Geometry check sheet. Reference: the model listing, model coordinates, mm. A direction names the side the tool comes from. Give positions to 0.01 mm unless a question says otherwise; leave off trailing zeros. Write each loop counter-clockwise with the first axis right and the second up, starting at its lowest first coordinate (ties: lowest second). Pieces come first, ordered by that corner, then holes. Notation, with made-up numbers: (-18, 81.5) - (37, 81.5) arc R10 cw to (37, 89.5) - close; hole circle Ø10 at (-37.75, -36.75). An arc over 180 degrees is marked (long way). Write item = value, one per line. Start each with the question number.
(1) Access from +Z, -Z, +X, -X, +Y, -Y to the whole of each face (thin tool, end or side, straight path). Record for faces 1 (the flat face through (-99, 1, 457.2)), 2 (the cylindrical face through (-62.084, 11.444, 392.811)).
(2) Section check C-C, the plane z = 399. Enter the section's corners in (x, y) (3 decimals), plus the area to 3 significant figures.
(3) Depth check by flat-ended pin: pin 1 Ø12 at (x, z) = (4, 264.5) entering from +Y; pin 2 Ø2 at (x, y) = (11.5, 147.5) entering from +Z; pin 3 Ø1.5 at (x, z) = (-137.5, 60.5) entering from +Y. Enter the tip coordinate at first touch or a pass-through.
(4) Section check A-A, the plane y = 0. Enter the section's corners in (x, z) (3 decimals), plus the area to 3 significant figures.
(5) Section check B-B, the plane x = 44.45. Enter the section's corners in (y, z), plus the area to 3 significant figures.
(6) Section check D-D, the plane z = 217.5. Enter the section's corners in (x, y).
(7) Thickness scan on L1, parallel to Z at x = 76, y = -124.5; L2, parallel to X at y = -14, z = 299.5; L3, parallel to Y at x = 138.5, z = 310.5. Record the ranges inside material, lowest first.
```python
from build123d import *

# Parameters (mm, degrees)
F1_DEPTH = 330.2
F2_R     = 38.1
F3_DEPTH = 127


with BuildPart() as f1:
    # F0 (on Top) → F1 (new body)
    with BuildSketch(Plane.XY):
        with BuildLine():
            Line((-216.284848, -72.686459), (-76.2, -171.332367))
            ThreePointArc((-76.2, -171.332367), (254, 0), (-76.2, 171.332367))
            Line((-76.2, 171.332367), (-216.284848, 72.686459))
            ThreePointArc((-216.284848, 72.686459), (-254, 0), (-216.284848, -72.686459))
        make_face()
    extrude(amount=F1_DEPTH)

    # F2 (on face) → F3 (join)
    with BuildSketch(Plane.XY.offset(330.2)):
        with Locations((-98.425, 0)):
            Circle(F2_R)
    extrude(amount=F3_DEPTH)


solid = f1.part
```
Model answer:
q1.face_1 = +Z, +X, -X, +Y, -Y
q1.face_2 = +Z
q2.outline = circle Ø76.2 at (-98.425, 0)
q2.area = 4,560 mm²
q3.pin_1 = 206.7
q3.pin_2 = 330.2
q3.pin_3 = 128.69
q4.outline = (-254, 0) - (254, 0) - (254, 330.2) - (-60.325, 330.2) - (-60.325, 457.2) - (-136.525, 457.2) - (-136.525, 330.2) - (-254, 330.2) - close
q4.area = 177,000 mm²
q5.outline = (-209.55, 0) - (209.55, 0) - (209.55, 330.2) - (-209.55, 330.2) - close
q5.area = 138,000 mm²
q6.outline = (-216.28, -72.69) - (-76.2, -171.33) arc R209.55 ccw (long way) to (-76.2, 171.33) - (-216.28, 72.69) arc R88.9 ccw to start
q7.L1 = 0 to 330.2
q7.L2 = -252.89 to 253.53
q7.L3 = -187.26 to 187.26
